Input: part model. Units: mm. Frame: model coordinates. A direction names the side the tool comes from. Coordinates: 2 decimals unless noted, no trailing zeros. Write each loop counter-clockwise with the first axis right and the second up, starting at its lowest first coordinate (ties: lowest second). Pieces come first, ordered by that corner, then holes. Notation, with made-up numbers: (62, 67) - (69, 67) arc R13 ccw to (69, 75) - close; hole circle Ø3 at (42.5, -5). An arc over 180 degrees is marked (long way). Use a Markdown table: item, result. Add a question column.
Q1. Section query A-A (x = -4.5). Return the cut outline in (y, z), then the cut area to 3 significant figures.
Q2. Material intervals for probe 1 along Z at (x, y) = (-0.25, 3.5); probe 2 along X at (y, z) = (-8.25, -1); probe 3 along Y at (x, z) = (-1.25, -7), sorted ascending. Write a range as from..to.
Q3. Section query B-B (z = -10.5). Return the cut outline in (x, y), then the cut area to 3 significant figures.
Q4. Set-up query: faces 4 (the face through (0, 0, -13)), 5 (the face through (0, -4, -11.5)), 6 (the face through (0.751, -10.972, 3.115)), 7 (the face through (0, 0, 13)), 8 (the face through (5, -5, 10)). Return all of +Z, -Z, +X, -X, +Y, -Y with unobstructed straight access to the full face (end or side cutting, diameter ignored); none if empty.
Q5. Pin query (flat end, axial travel): P1, Ø3, axis at x = -0.5, z = -13.5, coming from the +Y side; P2, Ø1, axis at x = -0.5, y = -8.5, coming from the +Z side; P3, Ø3, axis at x = 0.5, z = 14.5, coming from the -Y side. Return the tip coordinate at first contact, or that it passes through.
Q6. Mould query, pull axis Z, two halves, no side actions, for faces 1 (the face through (-0.046, -6.972, -2.636)), 2 (the face through (0, -4, 11.5)), 3 (the face through (-1, -9, 3)). Classes: released by +Z, released by -Z, zero draft, split by the parting line, or undercut.
from build123d import *

# Parameters (mm, degrees)
EXTRUDE_2_DEPTH      = 15
EXTRUDE_2_DEPTH_BACK = 5
SKETCH_1_W           = 12
SKETCH_1_H           = 23
EXTRUDE_3_DEPTH      = 4
SKETCH_3_R           = 2.5
EXTRUDE_4_DEPTH      = 4
SKETCH_4_W           = 12
SKETCH_4_H           = 4
EXTRUDE_5_DEPTH      = 2


with BuildPart() as part:
    # 草图1 → 凸台-拉伸2 (new, two sides: drawn at the far end of the back side and taken through both)
    with BuildSketch(Plane(origin=(0, 0, 0), x_dir=(1, 0, 0), z_dir=(0, 1, 0)).offset(-EXTRUDE_2_DEPTH_BACK)):
        Rectangle(SKETCH_1_W, SKETCH_1_H)
    extrude(amount=EXTRUDE_2_DEPTH + EXTRUDE_2_DEPTH_BACK)

    # 草图2 → 凸台-拉伸3 (add)
    with BuildSketch(Plane.XZ.offset(5)):
        with BuildLine():
            ThreePointArc((1.495922385, -0.310526329), (0, 11.5), (-1.495922385, -0.310526329))
            ThreePointArc((-1.495922385, -0.310526329), (0, -2.636784312), (1.495922385, -0.310526329))
        make_face()
    extrude(amount=EXTRUDE_3_DEPTH)

    # 草图3 → 凸台-拉伸4 (add)
    with BuildSketch(Plane.XZ.offset(9)):
        with Locations(Location((0, 5.5, 0), (0, 0, 270))):
            Circle(SKETCH_3_R)
    extrude(amount=EXTRUDE_4_DEPTH)

    # 草图4 → 凸台-拉伸5 (add)
    with BuildSketch(Plane(origin=(0, 0, 0), x_dir=(1, 0, 0), z_dir=(0, 1, 0))):
        with Locations((0, -13.5)):
            Rectangle(SKETCH_4_W, SKETCH_4_H)
    extrude_5 = extrude(amount=-EXTRUDE_5_DEPTH)

    # 镜向1: 凸台-拉伸5 across plane
    add(extrude_5.mirror(Plane.XY))


solid = part.part
Values follow:
| question | item | result |
|---|---|---|
| 1 | outline | (-9, 1.53) - (-5, 1.53) - (-5, -11.5) - (-2, -11.5) - (-2, -15.5) - (0, -15.5) - (0, -11.5) - (15, -11.5) - (15, 11.5) - (0, 11.5) - (0, 15.5) - (-2, 15.5) - (-2, 11.5) - (-5, 11.5) - (-5, 9.47) - (-9, 9.47) - close |
| 1 | area | 508 mm2 |
| 2 | probe 1 | -11.5..11.5 |
| 2 | probe 2 | -1.64..1.64 |
| 2 | probe 3 | -5..15 |
| 3 | outline | (-6, -5) - (6, -5) - (6, 15) - (-6, 15) - close |
| 3 | area | 240 mm2 |
| 4 | face 4 | -Z, +X, -X, +Y |
| 4 | face 5 | -Z, +X, -X, -Y |
| 4 | face 6 | -Y |
| 4 | face 7 | +Z, +X, -X, +Y |
| 4 | face 8 | +Z, +X, -Y |
| 5 | P1 | y = 0 |
| 5 | P2 | z = 11.5 |
| 5 | P3 | y = -2 |
| 6 | face 1 | undercut |
| 6 | face 2 | released by +Z |
| 6 | face 3 | zero draft |
